```python
from build123d import *

# Parameters (mm, degrees)
F0_W     = 50
F0_H     = 50
F1_DEPTH = 50
F2_R     = 17.5
F3_DEPTH = 50.001
F4_R     = 17.5
F5_DEPTH = 50.001
F6_R     = 17.5
F7_DEPTH = 50.001


with BuildPart() as f1:
    # F0 (on Front) → F1 (new body)
    with BuildSketch(Plane.XZ):
        Rectangle(F0_W, F0_H)
    extrude(amount=F1_DEPTH)

    # F2 (on face) → F3 (cut, through all)
    with BuildSketch(Plane.XZ.offset(50)):
        Circle(F2_R)
    extrude(amount=-F3_DEPTH, mode=Mode.SUBTRACT)

    # F4 (on face) → F5 (cut, through all)
    with BuildSketch(Plane.XY.offset(25)):
        with Locations((0, -25)):
            Circle(F4_R)
    extrude(amount=-F5_DEPTH, mode=Mode.SUBTRACT)

    # F6 (on face) → F7 (cut, through all)
    with BuildSketch(Plane.YZ.offset(25)):
        with Locations((-25, 0)):
            Circle(F6_R)
    extrude(amount=-F7_DEPTH, mode=Mode.SUBTRACT)


solid = f1.part
```
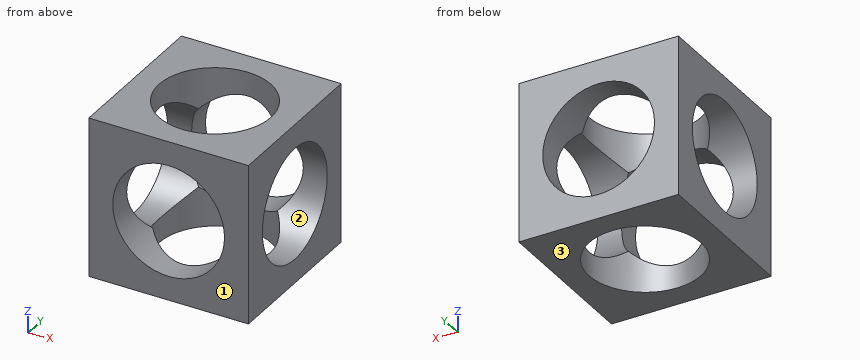
Model file for the job. Use its own axes, mm. Face numbers are marked on the shaded views. Give positions to 0.01 mm unless a question says otherwise; leave off trailing zeros. Write each loop counter-clockwise with the first axis right and the second up, starting at its lowest first coordinate (ties: lowest second). Pieces come first, ordered by that corner, then holes. Notation, with made-up numbers: M 55.25,83.5 L 85.25,83.5 A32 ccw 85.25,114.5 Z; hole C 66,68 d11. An arc over 180 degrees is marked long. Use a Markdown table: item, result.
1) Cut at A-A (z = 0). List the corners of the cut face in (x, y).
Responses:
| item | result |
|---|---|
| outline | M -25,-50 L -17.5,-50 L -17.5,-42.5 L -25,-42.5 Z; M -25,-7.5 L -17.5,-7.5 L -17.5,0 L -25,0 Z; M 17.5,-50 L 25,-50 L 25,-42.5 L 17.5,-42.5 Z; M 17.5,-7.5 L 25,-7.5 L 25,0 L 17.5,0 Z |
2) Drill centre lines: line 1 (X direction, y = -25, z = 21); line 2 (Y direction, x = 0, z = -18.5). Where is each one in solid material? Low to high. Write a range as from..to.
Responses:
| item | result |
|---|---|
| line 1 | x = -25..-17.5, 17.5..25 |
| line 2 | y = -50..-42.5, -7.5..0 |
3) Pin check, flat tip, straight feed: pin 1 (4 mm diameter, centred on y = -41, z = -1, fed in from -X). Stop position of the tip, or through.
Responses:
| item | result |
|---|---|
| pin 1 | stops at x = -25 |
4) Pull direction Z, two halves, no side cores. Call the marked faces 1, 2 and 3: +Z half, -Z half, draft (parallel to the pull), parting line (faces both ways), or undercut.
Responses:
| item | result |
|---|---|
| face 1 | draft |
| face 2 | undercut |
| face 3 | -Z half |
5) Cut at B-B (x = 0). List the corners of the cut face in (y, z).
Responses:
| item | result |
|---|---|
| outline | M -50,-25 L -42.5,-25 L -42.5,-17.5 L -50,-17.5 Z; M -50,17.5 L -42.5,17.5 L -42.5,25 L -50,25 Z; M -7.5,-25 L 0,-25 L 0,-17.5 L -7.5,-17.5 Z; M -7.5,17.5 L 0,17.5 L 0,25 L -7.5,25 Z |
6) Cut at D-D (x = 14). List the corners of the cut face in (y, z).
Responses:
| item | result |
|---|---|
| outline | M -50,-25 L -35.5,-25 L -35.5,-14 A17.5 cw -39,-10.5 L -50,-10.5 Z; M -50,10.5 L -39,10.5 A17.5 cw -35.5,14 L -35.5,25 L -50,25 Z; M -14.5,-25 L 0,-25 L 0,-10.5 L -11,-10.5 A17.5 cw -14.5,-14 Z; M -14.5,14 A17.5 cw -11,10.5 L 0,10.5 L 0,25 L -14.5,25 Z |
7) Cut at C-C (z = 20). List the corners of the cut face in (x, y), and give its area (3 significant figures).
Responses:
| item | result |
|---|---|
| outline | M -25,-50 L 25,-50 L 25,0 L -25,0 Z; hole C 0,-25 d35 |
| area | 1,540 mm2 |
